Source: CAD feature listing. Evaluate the final solid. Frame: model axes, mm. Round coordinates to 2 decimals unless told otherwise and drop trailing zeros. Loops run counter-clockwise (first coordinate to the right, second up) from the corner with the lowest first, then second, coordinate; pieces in that order, holes last. Notation, with made-up numbers: M 5,28.25 L 55,28.25 A15 cw 55,53.25 Z; hole C 86,32.25 d2. An arc over 180 degrees is marked long. One line per item, written item: value.
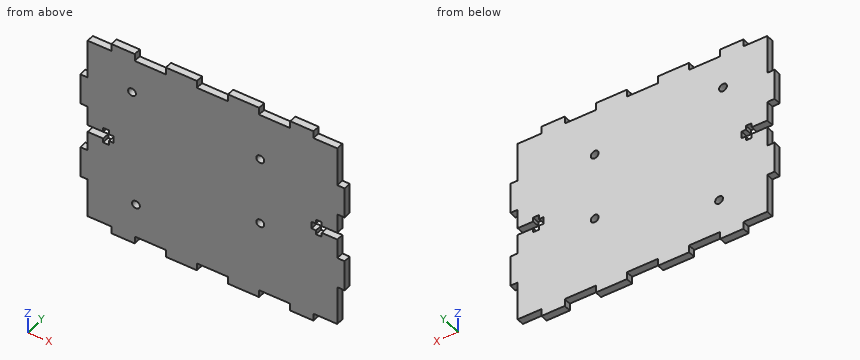
from build123d import *

# Parameters (mm, degrees)
SKETCH1_W           = 107.95
SKETCH1_H           = 82.55
BOSS_EXTRUDE1_DEPTH = 3
CUT_EXTRUDE2_REACH  = 137.929
SKETCH3_W           = 12.7
SKETCH3_H           = 3
SKETCH3_W_2         = 3
SKETCH3_H_2         = 19.05
CUT_EXTRUDE3_REACH  = 137.929
SKETCH4_R           = 1.6
CUT_EXTRUDE5_REACH  = 137.929


with BuildPart() as part:
    # Sketch1 → Boss-Extrude1 (new body)
    with BuildSketch(Plane(origin=(0, 0, 0), x_dir=(1, 0, 0), z_dir=(0, 1, 0))):
        with Locations((53.975, 41.275)):
            Rectangle(SKETCH1_W, SKETCH1_H)
    extrude(amount=BOSS_EXTRUDE1_DEPTH)

    # Sketch3 → Cut-Extrude2 (cut, up to next)
    with BuildSketch(Plane(origin=(0, 3, 0), x_dir=(1, 0, 0), z_dir=(0, 1, 0)), mode=Mode.PRIVATE) as cut_extrude2_sk1:
        with Locations((28.575, 1.5)):
            Rectangle(SKETCH3_W, SKETCH3_H)
    cut_extrude2_tool1 = extrude(cut_extrude2_sk1.sketch, amount=-CUT_EXTRUDE2_REACH, mode=Mode.PRIVATE) & part.part
    # Sketch3 → Cut-Extrude2 (cut, up to next)
    with BuildSketch(Plane(origin=(0, 3, 0), x_dir=(1, 0, 0), z_dir=(0, 1, 0)), mode=Mode.PRIVATE) as cut_extrude2_sk2:
        with Locations((79.375, 1.5)):
            Rectangle(SKETCH3_W, SKETCH3_H)
    cut_extrude2_tool2 = extrude(cut_extrude2_sk2.sketch, amount=-CUT_EXTRUDE2_REACH, mode=Mode.PRIVATE) & part.part
    # Sketch3 → Cut-Extrude2 (cut, up to next)
    with BuildSketch(Plane(origin=(0, 3, 0), x_dir=(1, 0, 0), z_dir=(0, 1, 0)), mode=Mode.PRIVATE) as cut_extrude2_sk3:
        with Locations((79.375, 81.05)):
            Rectangle(SKETCH3_W, SKETCH3_H)
    cut_extrude2_tool3 = extrude(cut_extrude2_sk3.sketch, amount=-CUT_EXTRUDE2_REACH, mode=Mode.PRIVATE) & part.part
    # Sketch3 → Cut-Extrude2 (cut, up to next)
    with BuildSketch(Plane(origin=(0, 3, 0), x_dir=(1, 0, 0), z_dir=(0, 1, 0)), mode=Mode.PRIVATE) as cut_extrude2_sk4:
        with Locations((1.5, 41.275)):
            Rectangle(SKETCH3_W_2, SKETCH3_H_2)
    cut_extrude2_tool4 = extrude(cut_extrude2_sk4.sketch, amount=-CUT_EXTRUDE2_REACH, mode=Mode.PRIVATE) & part.part
    # Sketch3 → Cut-Extrude2 (cut, up to next)
    with BuildSketch(Plane(origin=(0, 3, 0), x_dir=(1, 0, 0), z_dir=(0, 1, 0)), mode=Mode.PRIVATE) as cut_extrude2_sk5:
        with Locations((28.575, 81.05)):
            Rectangle(SKETCH3_W, SKETCH3_H)
    cut_extrude2_tool5 = extrude(cut_extrude2_sk5.sketch, amount=-CUT_EXTRUDE2_REACH, mode=Mode.PRIVATE) & part.part
    # Sketch3 → Cut-Extrude2 (cut, up to next)
    with BuildSketch(Plane(origin=(0, 3, 0), x_dir=(1, 0, 0), z_dir=(0, 1, 0)), mode=Mode.PRIVATE) as cut_extrude2_sk6:
        Polygon((53.975, 3), (60.325, 3), (60.325, 0), (53.975, 0), (47.625, 0), (47.625, 3), align=None)
    cut_extrude2_tool6 = extrude(cut_extrude2_sk6.sketch, amount=-CUT_EXTRUDE2_REACH, mode=Mode.PRIVATE) & part.part
    # Sketch3 → Cut-Extrude2 (cut, up to next)
    with BuildSketch(Plane(origin=(0, 3, 0), x_dir=(1, 0, 0), z_dir=(0, 1, 0)), mode=Mode.PRIVATE) as cut_extrude2_sk7:
        Polygon((60.325, 82.55), (53.975, 82.55), (47.625, 82.55), (47.625, 79.55), (53.975, 79.55), (60.325, 79.55), align=None)
    cut_extrude2_tool7 = extrude(cut_extrude2_sk7.sketch, amount=-CUT_EXTRUDE2_REACH, mode=Mode.PRIVATE) & part.part
    # Sketch3 → Cut-Extrude2 (cut, up to next)
    with BuildSketch(Plane(origin=(0, 3, 0), x_dir=(1, 0, 0), z_dir=(0, 1, 0)), mode=Mode.PRIVATE) as cut_extrude2_sk8:
        Polygon((0, 19.05), (3, 19.05), (3, 3), (12.7, 3), (12.7, 0), (0, 0), (0, 3), align=None)
    cut_extrude2_tool8 = extrude(cut_extrude2_sk8.sketch, amount=-CUT_EXTRUDE2_REACH, mode=Mode.PRIVATE) & part.part
    # Sketch3 → Cut-Extrude2 (cut, up to next)
    with BuildSketch(Plane(origin=(0, 3, 0), x_dir=(1, 0, 0), z_dir=(0, 1, 0)), mode=Mode.PRIVATE) as cut_extrude2_sk9:
        Polygon((107.95, 0), (107.95, 3), (107.95, 19.05), (104.95, 19.05), (104.95, 3), (95.25, 3), (95.25, 0), align=None)
    cut_extrude2_tool9 = extrude(cut_extrude2_sk9.sketch, amount=-CUT_EXTRUDE2_REACH, mode=Mode.PRIVATE) & part.part
    # Sketch3 → Cut-Extrude2 (cut, up to next)
    with BuildSketch(Plane(origin=(0, 3, 0), x_dir=(1, 0, 0), z_dir=(0, 1, 0)), mode=Mode.PRIVATE) as cut_extrude2_sk10:
        Polygon((0, 79.55), (0, 63.5), (3, 63.5), (3, 79.55), (12.7, 79.55), (12.7, 82.55), (0, 82.55), align=None)
    cut_extrude2_tool10 = extrude(cut_extrude2_sk10.sketch, amount=-CUT_EXTRUDE2_REACH, mode=Mode.PRIVATE) & part.part
    # Sketch3 → Cut-Extrude2 (cut, up to next)
    with BuildSketch(Plane(origin=(0, 3, 0), x_dir=(1, 0, 0), z_dir=(0, 1, 0)), mode=Mode.PRIVATE) as cut_extrude2_sk11:
        with Locations((106.45, 41.275)):
            Rectangle(SKETCH3_W_2, SKETCH3_H_2)
    cut_extrude2_tool11 = extrude(cut_extrude2_sk11.sketch, amount=-CUT_EXTRUDE2_REACH, mode=Mode.PRIVATE) & part.part
    # Sketch3 → Cut-Extrude2 (cut, up to next)
    with BuildSketch(Plane(origin=(0, 3, 0), x_dir=(1, 0, 0), z_dir=(0, 1, 0)), mode=Mode.PRIVATE) as cut_extrude2_sk12:
        Polygon((107.95, 63.5), (104.95, 63.5), (104.95, 79.55), (95.25, 79.55), (95.25, 82.55), (107.95, 82.55), (107.95, 79.55), align=None)
    cut_extrude2_tool12 = extrude(cut_extrude2_sk12.sketch, amount=-CUT_EXTRUDE2_REACH, mode=Mode.PRIVATE) & part.part
    add(cut_extrude2_tool1.solids().sort_by_distance((28.575, 3, -1.5))[0], mode=Mode.SUBTRACT)
    add(cut_extrude2_tool2.solids().sort_by_distance((79.375, 3, -1.5))[0], mode=Mode.SUBTRACT)
    add(cut_extrude2_tool3.solids().sort_by_distance((79.375, 3, -81.05))[0], mode=Mode.SUBTRACT)
    add(cut_extrude2_tool4.solids().sort_by_distance((1.5, 3, -41.275))[0], mode=Mode.SUBTRACT)
    add(cut_extrude2_tool5.solids().sort_by_distance((28.575, 3, -81.05))[0], mode=Mode.SUBTRACT)
    add(cut_extrude2_tool6.solids().sort_by_distance((53.975, 3, -1.5))[0], mode=Mode.SUBTRACT)
    add(cut_extrude2_tool7.solids().sort_by_distance((53.975, 3, -81.05))[0], mode=Mode.SUBTRACT)
    add(cut_extrude2_tool8.solids().sort_by_distance((1.5, 3, -18.821047))[0], mode=Mode.SUBTRACT)
    add(cut_extrude2_tool9.solids().sort_by_distance((107.721047, 3, -1.5))[0], mode=Mode.SUBTRACT)
    add(cut_extrude2_tool10.solids().sort_by_distance((0.228953, 3, -71.525))[0], mode=Mode.SUBTRACT)
    add(cut_extrude2_tool11.solids().sort_by_distance((106.45, 3, -41.275))[0], mode=Mode.SUBTRACT)
    add(cut_extrude2_tool12.solids().sort_by_distance((106.45, 3, -63.728953))[0], mode=Mode.SUBTRACT)

    # Sketch4 → Cut-Extrude3 (cut, up to next)
    with BuildSketch(Plane(origin=(0, 3, 0), x_dir=(1, 0, 0), z_dir=(0, 1, 0)), mode=Mode.PRIVATE) as cut_extrude3_sk1:
        with Locations(Location((22.6875, 65.425, 0), (0, 0, 270))):
            Circle(SKETCH4_R)
    cut_extrude3_tool1 = extrude(cut_extrude3_sk1.sketch, amount=-CUT_EXTRUDE3_REACH, mode=Mode.PRIVATE) & part.part
    # Sketch4 → Cut-Extrude3 (cut, up to next)
    with BuildSketch(Plane(origin=(0, 3, 0), x_dir=(1, 0, 0), z_dir=(0, 1, 0)), mode=Mode.PRIVATE) as cut_extrude3_sk2:
        with Locations(Location((21.0875, 17.125, 0), (0, 0, 270))):
            Circle(SKETCH4_R)
    cut_extrude3_tool2 = extrude(cut_extrude3_sk2.sketch, amount=-CUT_EXTRUDE3_REACH, mode=Mode.PRIVATE) & part.part
    # Sketch4 → Cut-Extrude3 (cut, up to next)
    with BuildSketch(Plane(origin=(0, 3, 0), x_dir=(1, 0, 0), z_dir=(0, 1, 0)), mode=Mode.PRIVATE) as cut_extrude3_sk3:
        with Locations(Location((73.4875, 22.225, 0), (0, 0, 270))):
            Circle(SKETCH4_R)
    cut_extrude3_tool3 = extrude(cut_extrude3_sk3.sketch, amount=-CUT_EXTRUDE3_REACH, mode=Mode.PRIVATE) & part.part
    # Sketch4 → Cut-Extrude3 (cut, up to next)
    with BuildSketch(Plane(origin=(0, 3, 0), x_dir=(1, 0, 0), z_dir=(0, 1, 0)), mode=Mode.PRIVATE) as cut_extrude3_sk4:
        with Locations(Location((73.4875, 50.125, 0), (0, 0, 270))):
            Circle(SKETCH4_R)
    cut_extrude3_tool4 = extrude(cut_extrude3_sk4.sketch, amount=-CUT_EXTRUDE3_REACH, mode=Mode.PRIVATE) & part.part
    add(cut_extrude3_tool1.solids().sort_by_distance((22.6875, 3, -65.425))[0], mode=Mode.SUBTRACT)
    add(cut_extrude3_tool2.solids().sort_by_distance((21.0875, 3, -17.125))[0], mode=Mode.SUBTRACT)
    add(cut_extrude3_tool3.solids().sort_by_distance((73.4875, 3, -22.225))[0], mode=Mode.SUBTRACT)
    add(cut_extrude3_tool4.solids().sort_by_distance((73.4875, 3, -50.125))[0], mode=Mode.SUBTRACT)

    # Sketch6 → Cut-Extrude5 (cut, up to next)
    with BuildSketch(Plane(origin=(0, 3, 0), x_dir=(1, 0, 0), z_dir=(0, 1, 0)), mode=Mode.PRIVATE) as cut_extrude5_sk1:
        Polygon((3, 39.8145), (9.35, 39.8145), (9.35, 38.0873), (11.6868, 38.0873), (11.6868, 39.8145), (13.49375, 39.8145), (13.49375, 41.275), (13.49375, 42.7355), (11.6868, 42.7355), (11.6868, 44.4627), (9.35, 44.4627), (9.35, 42.7355), (3, 42.7355), (3, 41.275), align=None)
    cut_extrude5_tool1 = extrude(cut_extrude5_sk1.sketch, amount=-CUT_EXTRUDE5_REACH, mode=Mode.PRIVATE) & part.part
    # Sketch6 → Cut-Extrude5 (cut, up to next)
    with BuildSketch(Plane(origin=(0, 3, 0), x_dir=(1, 0, 0), z_dir=(0, 1, 0)), mode=Mode.PRIVATE) as cut_extrude5_sk2:
        Polygon((94.45625, 42.7355), (94.45625, 41.275), (94.45625, 39.8145), (96.2632, 39.8145), (96.2632, 38.0873), (98.6, 38.0873), (98.6, 39.8145), (104.95, 39.8145), (104.95, 41.275), (104.95, 42.7355), (98.6, 42.7355), (98.6, 44.4627), (96.2632, 44.4627), (96.2632, 42.7355), align=None)
    cut_extrude5_tool2 = extrude(cut_extrude5_sk2.sketch, amount=-CUT_EXTRUDE5_REACH, mode=Mode.PRIVATE) & part.part
    add(cut_extrude5_tool1.solids().sort_by_distance((8.720382, 3, -41.275))[0], mode=Mode.SUBTRACT)
    add(cut_extrude5_tool2.solids().sort_by_distance((99.229618, 3, -41.275))[0], mode=Mode.SUBTRACT)


solid = part.part
1. Section query C-C (z = -5.5). Return the cut outline in (x, y), and give its area (3 significant figures).
Report:
outline: M 3,0 L 104.95,0 L 104.95,3 L 3,3 Z
area: 306 mm2
2. Section query B-B (x = 33). Return the cut outline in (y, z).
Report:
outline: M 0,-79.55 L 3,-79.55 L 3,-3 L 0,-3 Z
3. Ray query, line 1 (Z direction, x = 73.5, y = 0.9); line 2 (Z direction, x = 7, y = 0.8); line 3 (X direction, y = 0.55, z = -7). Return the intervals inside material, ascending. Write a range as [from, to].
Report:
line 1: z = [-79.55, -51.72], [-48.53, -23.82], [-20.63, -3]
line 2: z = [-79.55, -42.74], [-39.81, -3]
line 3: x = [3, 104.95]
4. Section query D-D (y = 1.45). Count the separate pieces of the cut face and the enclosed holes in it, and give its area (3 significant figures).
Report:
separate pieces: 1
enclosed holes: 4
area: 8,110 mm2
5. Pin query (flat end, axial travel): pin 1 (1.5 mm diameter, centred on y = 2, z = -1.5, fed in from -X); pin 2 (0.5 mm diameter, centred on y = 1.5, z = -39.5, fed in from -X); pin 3 (1.5 mm diameter, centred on y = 1, z = -13.5, fed in from +X). Return the tip coordinate at first contact, or that it passes through.
Report:
pin 1: stops at x = 12.7
pin 2: stops at x = 3
pin 3: stops at x = 104.95
6. Section query A-A (x = 101.5). Return the cut outline in (y, z), and give its area (3 significant figures).
Report:
outline: M 0,-79.55 L 3,-79.55 L 3,-42.74 L 0,-42.74 Z; M 0,-39.81 L 3,-39.81 L 3,-3 L 0,-3 Z
area: 221 mm2
